Job drawing, mm, ordinate dimensions from the low corner. One solid piece. Give positions to 0.01 mm unless a question says otherwise; leave off trailing zeros. Order: outer loops, then holes, each group sorted by start corner. A loop starts at its lowest first (then second) coordinate and runs counter-clockwise, first axis right, second up.
Item 1: Band-saw the part on B-B on x = 139.5. Give the cut face in (y, z).
Item 2: Wall check: L1, parallel to Y at x = 55, z = 2.05; L2, parallel to Y at x = 113, z = 7; L3, parallel to Z at x = 141, y = 95.5. Give the ranges that are in metal, low to high.
Item 3: Band-saw the part on C-C on z = 22. Give the cut face in (x, y), plus the area to 3 significant figures.
Item 4: Flat gauge pins, fed straight in: P1, Ø2, axis at y = 85, z = 30.5, coming from the +X side; P2, Ø5, axis at x = 139.5, y = 79, coming from the -Z side; P3, Ø4, axis at x = 153.5, z = 12.5, coming from the +Y side; P4, Ø3, axis at x = 132.5, z = 13, coming from the -Y side. Where does each tip first touch, or does it go through?
Item 5: Band-saw the part on A-A on y = 79. Give the cut face in (x, z).
Item 6: Band-saw the part on D-D on y = 134.5. Give the cut face in (x, z), plus the area to 3 significant figures.
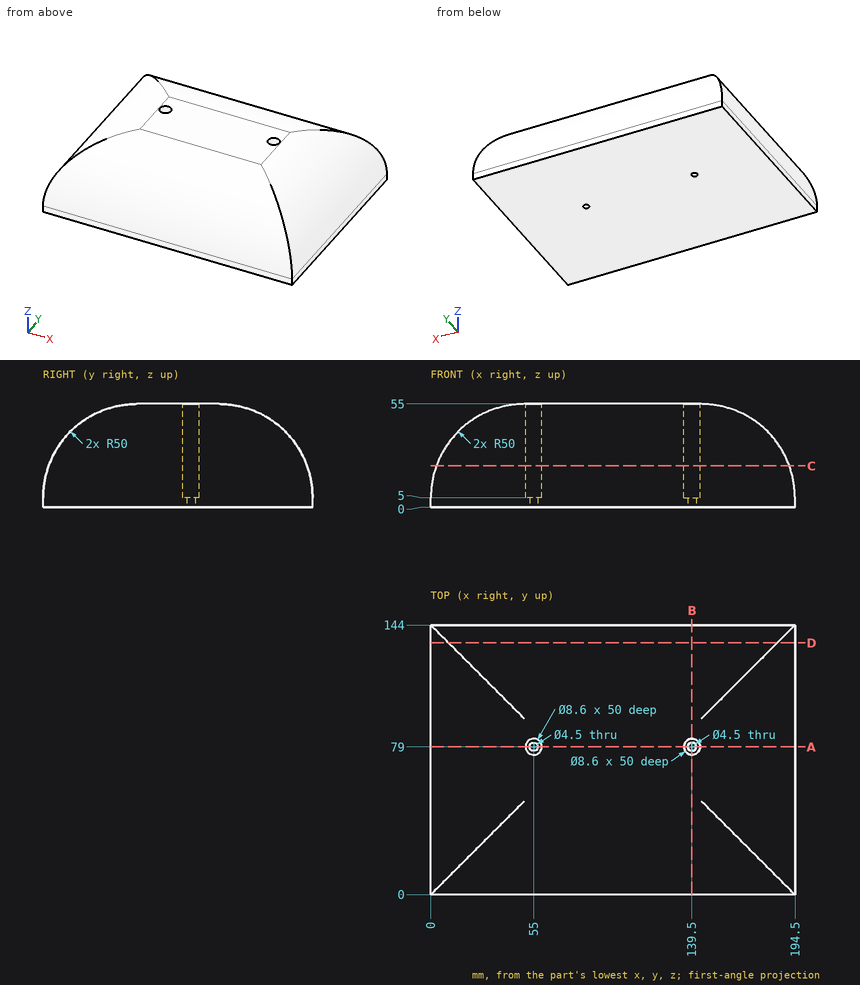
The answers:
1. outline: (0, 0) - (76.75, 0) - (76.75, 5) - (74.7, 5) - (74.7, 55) - (50, 55) arc R50 ccw to (0, 5) - close; (81.25, 0) - (144, 0) - (144, 5) arc R50 ccw to (94, 55) - (83.3, 55) - (83.3, 5) - (81.25, 5) - close
2. L1: y = 0 to 76.75, 81.25 to 144
2. L2: y = 0.04 to 143.96
2. L3: z = 0 to 54.98
3. outline: (2.98, 2.98) - (191.52, 2.98) - (191.52, 141.02) - (2.98, 141.02) - close; hole circle Ø8.6 at (55, 79); hole circle Ø8.6 at (139.5, 79)
3. area: 25,900 mm2
4. P1: stops at x = 188.09
4. P2: stops at z = 0
4. P3: stops at y = 143.7
4. P4: stops at y = 0.42
5. outline: (0, 0) - (52.75, 0) - (52.75, 5) - (50.7, 5) - (50.7, 55) - (50, 55) arc R50 ccw to (0, 5) - close; (57.25, 0) - (137.25, 0) - (137.25, 5) - (135.2, 5) - (135.2, 55) - (59.3, 55) - (59.3, 5) - (57.25, 5) - close; (141.75, 0) - (194.5, 0) - (194.5, 5) arc R50 ccw to (144.5, 55) - (143.8, 55) - (143.8, 5) - (141.75, 5) - close
6. outline: (0, 0) - (194.5, 0) - (194.5, 5) arc R50 ccw to (185, 34.32) - (9.5, 34.32) arc R50 ccw to (0, 5) - close
6. area: 6,500 mm2
